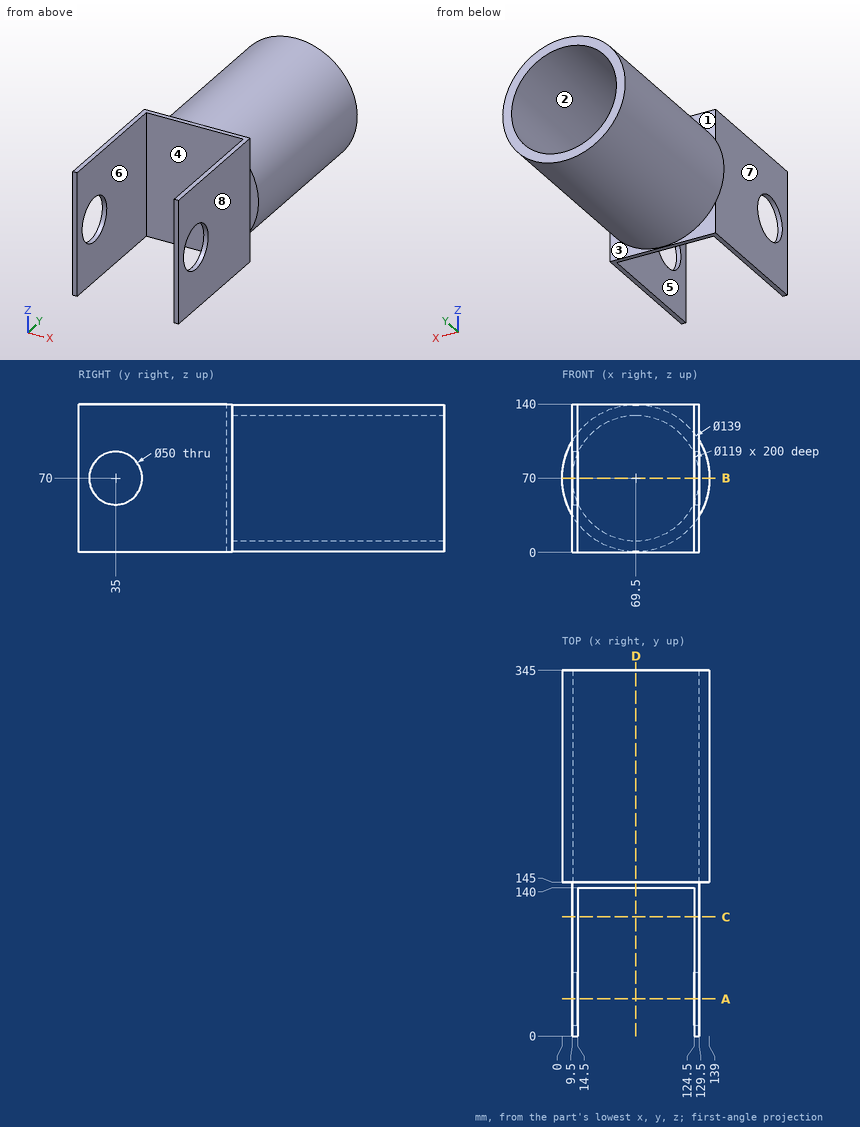
Print and shaded views of the part. All mm, measured from the part's lowest x, y and z. A direction names the side the tool comes from. Coordinates: 2 decimals unless noted, no trailing zeros. Write each loop counter-clockwise with the first axis right and the second up, starting at its lowest first coordinate (ties: lowest second). Pieces come first, ordered by that corner, then holes.
(1) Cut at B-B, the plane z = 70. List the corners of the cut face in (x, y).
(2) 3-axis set-ups, long thin cutter, end or side, ignore diameter. For the marked faces 1, 2, 3 and 4: which of +Z, -Z, +X, -X, +Y, -Y reach the whole face in a straight line?
(3) Cut at A-A, the plane y = 35. List the corners of the cut face in (x, z).
(4) Cut at C-C, the plane y = 112.5. List the corners of the cut face in (x, z).
(5) Two-plate mould, pull along X, no slides. Class the marked faces 5, 6, 7 and 8: +X half, -X half, draft (parallel to the pull), parting line (faces both ways), or undercut.
(6) Flat gauge pins, fed straight in: pin 1 (17.5 mm diameter, centred on x = 51, z = 115.5, fed in from +Y); pin 2 (2 mm diameter, centred on x = 44.5, z = 72, fed in from -Y); pin 3 (10.5 mm diameter, centred on x = 135, z = 77, fed in from -Y). Where does each tip first touch, or does it go through?
(7) Drill centre lines: probe 1 along X at (y, z) = (85, 55.5); probe 2 along Y at (x, z) = (12.2, 70); probe 3 along Z at (x, y) = (11.1, 35). Where is each one in solid material? Low to high.
(8) Cut at D-D, the plane x = 69.5. List the corners of the cut face in (y, z), and give its area (3 significant figures).
Geometry says:
1. outline: (0, 145) - (9.5, 145) - (9.5, 60) - (14.5, 60) - (14.5, 140) - (124.5, 140) - (124.5, 60) - (129.5, 60) - (129.5, 145) - (139, 145) - (139, 345) - (129, 345) - (129, 145) - (10, 145) - (10, 345) - (0, 345) - close; (9.5, 0) - (14.5, 0) - (14.5, 10) - (9.5, 10) - close; (124.5, 0) - (129.5, 0) - (129.5, 10) - (124.5, 10) - close
2. face 1: +Z, +Y
2. face 2: +Y
2. face 3: -Z, +Y
2. face 4: +Z, -Z, -Y
3. outline: (9.5, 0) - (14.5, 0) - (14.5, 45) - (9.5, 45) - close; (9.5, 95) - (14.5, 95) - (14.5, 140) - (9.5, 140) - close; (124.5, 0) - (129.5, 0) - (129.5, 45) - (124.5, 45) - close; (124.5, 95) - (129.5, 95) - (129.5, 140) - (124.5, 140) - close
4. outline: (9.5, 0) - (14.5, 0) - (14.5, 140) - (9.5, 140) - close; (124.5, 0) - (129.5, 0) - (129.5, 140) - (124.5, 140) - close
5. face 5: undercut
5. face 6: undercut
5. face 7: -X half
5. face 8: +X half
6. pin 1: stops at y = 145
6. pin 2: stops at y = 140
6. pin 3: stops at y = 145
7. probe 1: x = 9.5 to 14.5, 124.5 to 129.5
7. probe 2: y = 0 to 10, 60 to 145
7. probe 3: z = 0 to 45, 95 to 140
8. outline: (140, 0) - (145, 0) - (145, 0.5) - (345, 0.5) - (345, 10.5) - (145, 10.5) - (145, 129.5) - (345, 129.5) - (345, 139.5) - (145, 139.5) - (145, 140) - (140, 140) - close
8. area: 4,700 mm2
